from build123d import *

# Parameters (mm, degrees)
SKETCH_1_R          = 5
SKETCH_1_R_2        = 1.55
EXTRUDE_1_DEPTH     = 4.75
SKETCH_2_R          = 2.75
SKETCH_2_R_2        = 1.55
EXTRUDE_2_DEPTH     = 2
CUT_EXTRUDE_1_DEPTH = 2.75


with BuildPart() as part:
    # 草图1 → 凸台-拉伸1 (new body)
    with BuildSketch(Plane.XY):
        Circle(SKETCH_1_R)
        Circle(SKETCH_1_R_2, mode=Mode.SUBTRACT)
    extrude(amount=EXTRUDE_1_DEPTH)

    # 草图2 → 凸台-拉伸2 (add)
    with BuildSketch(Plane.XY.offset(4.75)):
        Circle(SKETCH_2_R)
        Circle(SKETCH_2_R_2, mode=Mode.SUBTRACT)
    extrude(amount=EXTRUDE_2_DEPTH)

    # 草图3 → 切除-拉伸1 (cut)
    with BuildSketch(Plane(origin=(0, 0, 0), x_dir=(-1, 0, 0), z_dir=(0, 0, -1))):
        Polygon((1.770357817, 2.977554903), (-1.693459279, 3.021952295), (-3.463817096, 0.044397392), (-1.770357817, -2.977554903), (1.693459279, -3.021952295), (3.463817096, -0.044397392), align=None)
    extrude(amount=-CUT_EXTRUDE_1_DEPTH, mode=Mode.SUBTRACT)


solid = part.part
Can you work these out from the model? Positions are in its coordinate system, mm. A direction names the side the tool comes from. Give positions to 0.01 mm unless a question says otherwise; leave off trailing zeros. Loops run counter-clockwise (first coordinate to the right, second up) from the corner with the lowest first, then second, coordinate; pieces in that order, holes last. Notation, with made-up numbers: (33.5, 75.25) -> (60.5, 75.25) arc R13 cw to (60.5, 79.25) -> close; hole circle Ø9 at (-28, -20). An arc over 180 degrees is marked (long way). Use one line per item in the form item = value.
1) Will these pins go through, and if not, where does the flat tip stop? pin 1 (3 mm diameter, centred on y = 3, z = 3, fed in from +X); pin 2 (5 mm diameter, centred on x = 0, y = 0, fed in from -Z).
Answers:
pin_1 = 4.77
pin_2 = 2.75
2) If we section it at B-B (y = -1.25): Please give me the cut outline in (x, z), plus the area to 3 significant figures.
Answers:
outline = (-4.84, 0) -> (-2.75, 0) -> (-2.75, 2.75) -> (-0.92, 2.75) -> (-0.92, 6.75) -> (-2.45, 6.75) -> (-2.45, 4.75) -> (-4.84, 4.75) -> close; (0.92, 2.75) -> (2.74, 2.75) -> (2.74, 0) -> (4.84, 0) -> (4.84, 4.75) -> (2.45, 4.75) -> (2.45, 6.75) -> (0.92, 6.75) -> close
area = 33.4 mm²
3) For faces 4 (the face through (2.2, -2.2, 4.75)), 5 (the face through (-2.629, 1.445, 1.356)), 6 (the face through (-0.1, -3.3, 0)), which set-ups out of +Z, -Z, +X, -X, +Y, -Y let a thin tool reach every point of the face, with its end or its side?
Answers:
face_4 = +Z
face_5 = -Z
face_6 = -Z, +X, -X, +Y, -Y
4) If we section it at C-C (x = 3.25): Please give me the cut outline in (y, z).
Answers:
outline = (-3.8, 0) -> (-0.34, 0) -> (-0.34, 2.75) -> (0.4, 2.75) -> (0.4, 0) -> (3.8, 0) -> (3.8, 4.75) -> (-3.8, 4.75) -> close
5) I need wall thicknesses on line 1 along Y through (x, z) = (0, 4.5); line 2 along Y through (x, z) = (0, 5.9); line 3 along Z through (x, y) = (3.25, 0). Which ranges of each line are inside material? Lowest first, please.
Answers:
line_1 = -5 to -1.55, 1.55 to 5
line_2 = -2.75 to -1.55, 1.55 to 2.75
line_3 = 2.75 to 4.75
6) We'd pull the mould along X, two halves only. Please class faces 1 (the face through (2, 0, 2.75)), 2 (the face through (-0.596, -2.685, 5.736)), 3 (the face through (2, 0, 6.75)): released by +X, released by -X, zero draft, split by the parting line, or undercut.
Answers:
face_1 = undercut
face_2 = split by the parting line
face_3 = zero draft
7) If we section it at D-D (z = 5.75): Please give me the cut outline in (x, y), plus the area to 3 significant figures.
Answers:
outline = circle Ø5.5 at (0, 0); hole circle Ø3.1 at (0, 0)
area = 16.2 mm²
8) If we section it at A-A (x = 0.5): Please give me the cut outline in (y, z).
Answers:
outline = (-4.97, 0) -> (-2.99, 0) -> (-2.99, 2.75) -> (-1.47, 2.75) -> (-1.47, 6.75) -> (-2.7, 6.75) -> (-2.7, 4.75) -> (-4.97, 4.75) -> close; (1.47, 2.75) -> (3.01, 2.75) -> (3.01, 0) -> (4.97, 0) -> (4.97, 4.75) -> (2.7, 4.75) -> (2.7, 6.75) -> (1.47, 6.75) -> close
